Could you check a few things on this model? Use its own coordinates, in mm. Face numbers are marked on the shaded views. A direction names the side the tool comes from. Give positions to 0.01 mm unless a question says otherwise; leave off trailing zeros. Loops run counter-clockwise (first coordinate to the right, second up) from the corner with the lowest first, then second, coordinate; pieces in that order, holes last. Notation, with made-up numbers: M 4.25,-6.75 L 48.25,-6.75 A6 ccw 48.25,-1.75 Z; hole C 45.5,-14 d7. An arc over 180 degrees is marked long. Use a Markdown table: item, result. Add a question column.
1) Suppose I cut it at A-A on x = 52. List the corners of the cut face in (y, z) for me.
2) Suppose I cut it at D-D on z = 24.75. Count the separate pieces of the cut face and the enclosed holes in it, and give its area (3 significant figures).
3) Which directions (+Z, -Z, +X, -X, +Y, -Y) give clear straight access to the entire face, cutting with the end or side of a thin tool? Please do the marked faces 1, 2, 3, 4 and 5.
4) If I drill on line 1 along Z through (x, y) = (26.75, 1.75); line 2 along X through (y, z) = (3.25, -6.75); line 3 along X through (y, z) = (2, -6), over which ranges is the centre line in solid material (lowest first)? Write a range as [from, to].
5) Will these pins go through, and if not, where does the flat tip stop? pin 1 Ø4.5 at (x, z) = (26.75, -6.75) entering from +Y; pin 2 Ø6.5 at (x, z) = (-26.75, 24.75) entering from -Y; pin 3 Ø8 at (x, z) = (29, 20) entering from -Y; pin 4 Ø4 at (x, z) = (-56.5, -17) entering from +Y.
6) Suppose I cut it at B-B on y = -9. List the corners of the cut face in (x, z) for me.
7) We'd pull the mould along X, two halves only. Please class the marked faces 6, 7 and 8: +X half, -X half, draft (parallel to the pull), parting line (faces both ways), or undercut.
8) Suppose I cut it at C-C on z = 2.5. List the corners of the cut face in (x, y) for me, and give its area (3 significant figures).
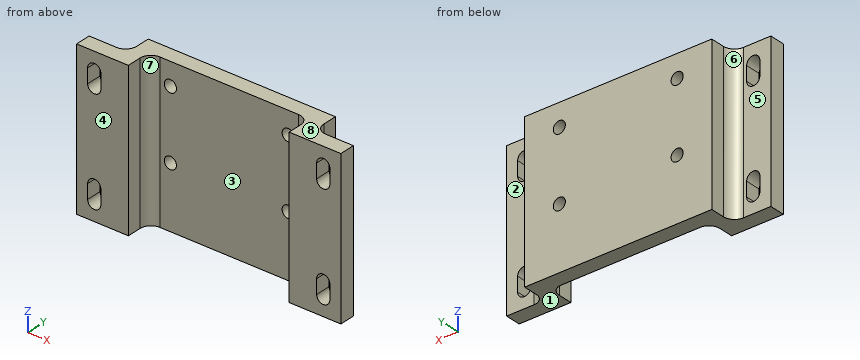
```python
from build123d import *

# Parameters (mm, degrees)
BOSS_EXTRUDE1_DEPTH      = 35
BOSS_EXTRUDE1_DEPTH_BACK = 35
FILLET1_R                = 5
CUT_EXTRUDE1_DEPTH       = 71.407741052
CUT_EXTRUDE1_DEPTH_BACK  = 71.407741052
SKETCH2_R                = 3
SKETCH2_R_2              = 2.75


with BuildPart() as part:
    # Sketch1 → Boss-Extrude1 (new, two sides: drawn at the far end of the back side and taken through both)
    with BuildSketch(Plane.XY.offset(-BOSS_EXTRUDE1_DEPTH_BACK)):
        Polygon((-60, -11.5), (-36.5, -11.5), (-36.5, 0), (36.5, 0), (36.5, -11.5), (60, -11.5), (60, -4.5), (42.5, -4.5), (42.5, 7), (-42.5, 7), (-42.5, -4.5), (-60, -4.5), align=None)
    extrude(amount=BOSS_EXTRUDE1_DEPTH + BOSS_EXTRUDE1_DEPTH_BACK)

    # Fillet1
    fillet1_edges = [part.edges().sort_by_distance(p)[0] for p in [
        (-42.5, -4.5, 0),
        (42.5, -4.5, 0),
        (36.5, 0, 0),
        (-36.5, 0, 0),
    ]]
    fillet(fillet1_edges, radius=FILLET1_R)

    # Sketch2 → Cut-Extrude1 (cut, two sides: drawn at the far end of the back side and taken through both)
    with BuildSketch(Plane(origin=(0, 0, 0), x_dir=(1, 0, 0), z_dir=(0, 1, 0)).offset(-CUT_EXTRUDE1_DEPTH_BACK)):
        with Locations((-52, 27)):
            Circle(SKETCH2_R)
        with BuildLine():
            ThreePointArc((-49, 27), (-52, 24), (-55, 27))
            Line((-55, 27), (-55, 20.5))
            ThreePointArc((-55, 20.5), (-52, 23.5), (-49, 20.5))
            Line((-49, 20.5), (-49, 27))
        make_face()
        with Locations((-52, 20.5)):
            Circle(SKETCH2_R)
        with Locations((-52, -20.5)):
            Circle(SKETCH2_R)
        with BuildLine():
            ThreePointArc((-49, -20.5), (-52, -23.5), (-55, -20.5))
            Line((-55, -20.5), (-55, -27))
            ThreePointArc((-55, -27), (-52, -24), (-49, -27))
            Line((-49, -27), (-49, -20.5))
        make_face()
        with Locations((-52, -27)):
            Circle(SKETCH2_R)
        with Locations((52, -20.5)):
            Circle(SKETCH2_R)
        with BuildLine():
            Line((55, -27), (55, -20.5))
            ThreePointArc((55, -20.5), (52, -23.5), (49, -20.5))
            Line((49, -20.5), (49, -27))
            ThreePointArc((49, -27), (52, -24), (55, -27))
        make_face()
        with Locations((52, -27)):
            Circle(SKETCH2_R)
        with Locations((52, 27)):
            Circle(SKETCH2_R)
        with BuildLine():
            Line((55, 20.5), (55, 27))
            ThreePointArc((55, 27), (52, 24), (49, 27))
            Line((49, 27), (49, 20.5))
            ThreePointArc((49, 20.5), (52, 23.5), (55, 20.5))
        make_face()
        with Locations((52, 20.5)):
            Circle(SKETCH2_R)
        with Locations(Location((-26.75, 6.75, 0), (0, 0, 270))):
            Circle(SKETCH2_R_2)
        with Locations(Location((26.75, 6.75, 0), (0, 0, 270))):
            Circle(SKETCH2_R_2)
        with Locations(Location((26.75, -24.75, 0), (0, 0, 270))):
            Circle(SKETCH2_R_2)
        with Locations(Location((-26.75, -24.75, 0), (0, 0, 270))):
            Circle(SKETCH2_R_2)
    extrude(amount=CUT_EXTRUDE1_DEPTH + CUT_EXTRUDE1_DEPTH_BACK, mode=Mode.SUBTRACT)


solid = part.part
```
Answer block:
| question | item | result |
|---|---|---|
| 1 | outline | M -11.5,-35 L -4.5,-35 L -4.5,-30 L -11.5,-30 Z; M -11.5,-17.5 L -4.5,-17.5 L -4.5,17.5 L -11.5,17.5 Z; M -11.5,30 L -4.5,30 L -4.5,35 L -11.5,35 Z |
| 2 | separate pieces | 5 |
| 2 | enclosed holes | 0 |
| 2 | area | 838 mm^2 |
| 3 | face 1 | -Z, +X, -X, +Y, -Y |
| 3 | face 2 | +Z, -Z, +X, +Y |
| 3 | face 3 | +Z, -Z, -Y |
| 3 | face 4 | +Z, -Z, +X, -X, -Y |
| 3 | face 5 | +Z, -Z, -X, +Y |
| 4 | line 1 | z = [-35, -9.5], [-4, 22], [27.5, 35] |
| 4 | line 2 | x = [-42.5, -29.5], [-24, 24], [29.5, 42.5] |
| 4 | line 3 | x = [-42.5, -29.4], [-24.1, 24.1], [29.4, 42.5] |
| 5 | pin 1 | passes through |
| 5 | pin 2 | stops at y = 0 |
| 5 | pin 3 | stops at y = -0.23 |
| 5 | pin 4 | stops at y = -4.5 |
| 6 | outline | M -60,-35 L -36.5,-35 L -36.5,35 L -60,35 Z; M 36.5,-35 L 60,-35 L 60,35 L 36.5,35 Z; hole M -55,-27 A3 ccw -49,-27 L -49,-20.5 A3 ccw -55,-20.5 Z; hole M -55,20.5 A3 ccw -49,20.5 L -49,27 A3 ccw -55,27 Z; hole M 49,-27 A3 ccw 55,-27 L 55,-20.5 A3 ccw 49,-20.5 Z; hole M 49,20.5 A3 ccw 55,20.5 L 55,27 A3 ccw 49,27 Z |
| 7 | face 6 | -X half |
| 7 | face 7 | undercut |
| 7 | face 8 | draft |
| 8 | outline | M -60,-11.5 L -36.5,-11.5 L -36.5,-5 A5 cw -31.5,0 L 31.5,0 A5 cw 36.5,-5 L 36.5,-11.5 L 60,-11.5 L 60,-4.5 L 47.5,-4.5 A5 cw 42.5,0.5 L 42.5,7 L -42.5,7 L -42.5,0.5 A5 cw -47.5,-4.5 L -60,-4.5 Z |
| 8 | area | 999 mm^2 |
